Geometry: final body of the model. Coordinates: model frame, mm. Round coordinates to 2 decimals unless told otherwise and drop trailing zeros. Order: outer loops, then holes, each group sorted by start corner. A loop starts at its lowest first (then second) coordinate and runs counter-clockwise, first axis right, second up. Notation, with made-up numbers: M 22,65.5 L 69,65.5 A14 ccw 69,91.5 Z; hole C 59,0 d3. An arc over 180 degrees is marked long. Return JSON: item names as keys, results as strings. Group by question number.
Q1. Cut plane A-A on x = 43. Output: boundary loops of the cut face in (y, z), and give its area (3 significant figures).
Q2. Cut plane C-C on z = 380. Output: boundary loops of the cut face in (x, y).
Q3. Ray query, probe 1 along Z at (x, y) = (52.5, -23.5); probe 2 along Z at (x, y) = (45.5, -12.7); probe 3 along X at (y, z) = (-4.5, 61) (3 decimals). Return the intervals inside material, ascending.
Q4. Cut plane B-B on y = -12.7. Count the separate pieces of the cut face and the enclosed holes in it, and give its area (3 significant figures).
```python
from build123d import *

# Parameters (mm, degrees)
F0_W     = 76.2
F0_H     = 400
F1_DEPTH = 25.4
F3_D     = 17.5
F4_W     = 57.15
F4_H     = 76.2
F4_H_2   = 44.45
F5_DEPTH = 25.401
F6_R     = 5.08
F7_R     = 5.08


with BuildPart() as f1:
    # F0 (on Front) → F1 (new body)
    with BuildSketch(Plane.XZ):
        with Locations((38.1, 200)):
            Rectangle(F0_W, F0_H)
    extrude(amount=F1_DEPTH)

    # F3 (through all)
    with Locations(Plane.YZ.offset(76.2)):
        with Locations((-12.7, 380), (-12.7, 20)):
            Hole(F3_D / 2)

    # F4 (on face) → F5 (cut, through all)
    with BuildSketch(Plane.XZ.offset(25.4)):
        with Locations((38.1, 70.1)):
            Rectangle(F4_W, F4_H)
        with Locations((38.1, 345.775)):
            Rectangle(F4_W, F4_H_2)
    extrude(amount=-F5_DEPTH, mode=Mode.SUBTRACT)

    # F6
    f6_edges = [f1.edges().sort_by_distance(p)[0] for p in [
        (9.525, -12.7, 108.2),
        (66.675, -12.7, 108.2),
        (66.675, -12.7, 32),
        (9.525, -12.7, 32),
        (9.525, -12.7, 323.55),
        (66.675, -12.7, 323.55),
        (9.525, -12.7, 368),
        (66.675, -12.7, 368),
    ]]
    fillet(f6_edges, radius=F6_R)

    # F7
    f7_edges = [f1.edges().sort_by_distance(p)[0] for p in [
        (76.2, -12.7, 400),
    ]]
    fillet(f7_edges, radius=F7_R)


solid = f1.part
```
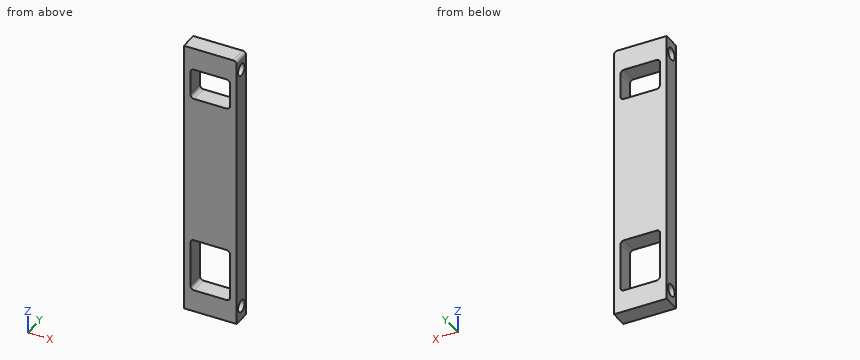
Result sheet:
{
 "1": {"outline": "M -25.4,0 L 0,0 L 0,32 L -25.4,32 Z; M -25.4,108.2 L 0,108.2 L 0,323.55 L -25.4,323.55 Z; M -25.4,368 L 0,368 L 0,400 L -25.4,400 Z; hole C -12.7,20 d17.5; hole C -12.7,380 d17.5", "area": "6,610 mm²"},
 "2": {"outline": "M 0,-25.4 L 76.2,-25.4 L 76.2,-21.45 L 0,-21.45 Z; M 0,-3.95 L 76.2,-3.95 L 76.2,0 L 0,0 Z"},
 "3": {"probe 1": "z = 0 to 32, 108.2 to 323.55, 368 to 400", "probe 2": "z = 0 to 11.25, 28.75 to 32, 108.2 to 323.55, 368 to 371.25, 388.75 to 400", "probe 3": "x = 0 to 9.525, 66.675 to 76.2"},
 "4": {"separate pieces": "3", "enclosed holes": "2", "area": "21,000 mm²"}
}
